from build123d import *

# Parameters (mm, degrees)
BOSS_EXTRUDE1_DEPTH = 3.175
FILLET1_R           = 4.7625
SKETCH2_R           = 6.35
CUT_EXTRUDE1_DEPTH  = 36.892950213


with BuildPart() as part:
    # Sketch1 → Boss-Extrude1 (new body)
    with BuildSketch(Plane(origin=(0, 0, 0), x_dir=(1, 0, 0), z_dir=(0, 1, 0))):
        with BuildLine():
            ThreePointArc((-4.826, 11.057755152), (0, -12.065), (4.826, 11.057755152))
            Line((4.826, 11.057755152), (4.826, 33.655))
            Line((4.826, 33.655), (-4.826, 33.655))
            Line((-4.826, 33.655), (-4.826, 11.057755152))
        make_face()
    extrude(amount=BOSS_EXTRUDE1_DEPTH)

    # Fillet1
    fillet1_edges = [part.edges().sort_by_distance(p)[0] for p in [
        (4.826, 1.5875, -11.057755152),
        (-4.826, 1.5875, -11.057755152),
        (-4.826, 1.5875, -33.655),
        (4.826, 1.5875, -33.655),
    ]]
    fillet(fillet1_edges, radius=FILLET1_R)

    # Sketch2 → Cut-Extrude1 (cut, through all)
    with BuildSketch(Plane(origin=(0, 3.175, 0), x_dir=(1, 0, 0), z_dir=(0, 1, 0))):
        with Locations(Location((0, 0, 0), (0, 0, 270))):
            Circle(SKETCH2_R)
    extrude(amount=-CUT_EXTRUDE1_DEPTH, mode=Mode.SUBTRACT)


solid = part.part
Verification items for the finished model (mm, model axes). A direction names the side the tool comes from. Round coordinates to 2 decimals unless told otherwise and drop trailing zeros. Order: outer loops, then holes, each group sorted by start corner. A loop starts at its lowest first (then second) coordinate and runs counter-clockwise, first axis right, second up. Notation, with made-up numbers: (66, 70) -> (79, 70) arc R18 ccw to (79, 100) -> close; hole circle Ø5 at (-12.75, -38.5). An arc over 180 degrees is marked (long way). Put each result on its own line as item: value.
1) Section check B-B (x = 1.75). Record the cut outline in (y, z) (3 decimals).
Final values:
outline: (0, -33.346) -> (3.175, -33.346) -> (3.175, -6.104) -> (0, -6.104) -> close; (0, 6.104) -> (3.175, 6.104) -> (3.175, 11.937) -> (0, 11.937) -> close
2) Material ranges on line 1 (X direction, y = 1.55, z = 0) (3 decimals); line 2 (X direction, y = 2.55, z = -15.5); line 3 (X direction, y = 1.9, z = 5.5), recorded low to high.
Final values:
line 1: x = -12.065 to -6.35, 6.35 to 12.065
line 2: x = -4.83 to 4.83
line 3: x = -10.74 to -3.17, 3.17 to 10.74
3) Depth check by flat-ended pin: pin 1 (1 mm diameter, centred on y = 1, z = 4, fed in from +X); pin 2 (1.5 mm diameter, centred on y = 2, z = -7, fed in from -X); pin 3 (1 mm diameter, centred on y = 1, z = -12, fed in from +X). Enter the tip coordinate at first touch or a pass-through.
Final values:
pin 1: stops at x = 11.55
pin 2: stops at x = -10.32
pin 3: stops at x = 5.43
4) Mould release check, pull along Z, two halves, no side actions. Record for faces 1 (the cylindrical face through (5.384, 1.61, -11.591)), 2 (the cylindrical face through (-3.86, 1.61, -5.04)), 3 (the flat face through (4.826, 2, -21)): +Z half, -Z half, draft (parallel to the pull), parting line (faces both ways), or undercut.
Final values:
face 1: -Z half
face 2: undercut
face 3: draft
5) Section check A-A (z = 0). Record the cut outline in (x, y) (3 decimals).
Final values:
outline: (-12.065, 0) -> (-6.35, 0) -> (-6.35, 3.175) -> (-12.065, 3.175) -> close; (6.35, 0) -> (12.065, 0) -> (12.065, 3.175) -> (6.35, 3.175) -> close
6) Set-up check for faces 4 (the flat face through (-4.826, 2, -21)), 5 (the cylindrical face through (-0.428, 1.565, 12.057)): record each of +Z, -Z, +X, -X, +Y, -Y from which the full face is reachable in a straight line by a thin tool's end or side.
Final values:
face 4: -Z, -X, +Y, -Y
face 5: +Y, -Y
7) Section check D-D (x = 8.5). Record the cut outline in (y, z) (3 decimals).
Final values:
outline: (0, -8.562) -> (3.175, -8.562) -> (3.175, 8.562) -> (0, 8.562) -> close
